Check sheet for the drawn part. Datum: minimum x, y, z corner. Units: mm. Round coordinates to 2 decimals unless told otherwise and drop trailing zeros. Write each loop counter-clockwise with the first axis right and the second up, starting at its lowest first coordinate (ties: lowest second). Pieces come first, ordered by that corner, then holes.
Item 1: Cross-section at A-A on z = 161. Enter the section's corners in (x, y).
Item 2: Material ranges on line 1 (X direction, y = 2.55, z = 169); line 2 (Z direction, x = 19.5, y = 2.7), recorded low to high.
Item 3: Go/stop test with flat-tipped pins: pin 1 Ø1.5 at (x, y) = (75.5, 2) entering from +Z; pin 2 Ø1.5 at (y, z) = (2, 165) entering from -X; pin 3 Ø4 at (x, z) = (132, 134.5) entering from +Y; pin 4 Ø8 at (x, z) = (129, 112) entering from -Y. Record where each tip stops, or that it passes through.
Item 4: Cross-section at B-B on y = 1.3. Enter the section's corners in (x, z), plus the area to 3 significant figures.
Item 5: Cross-section at C-C on x = 31.5. Enter the section's corners in (y, z), plus the area to 3 significant figures.
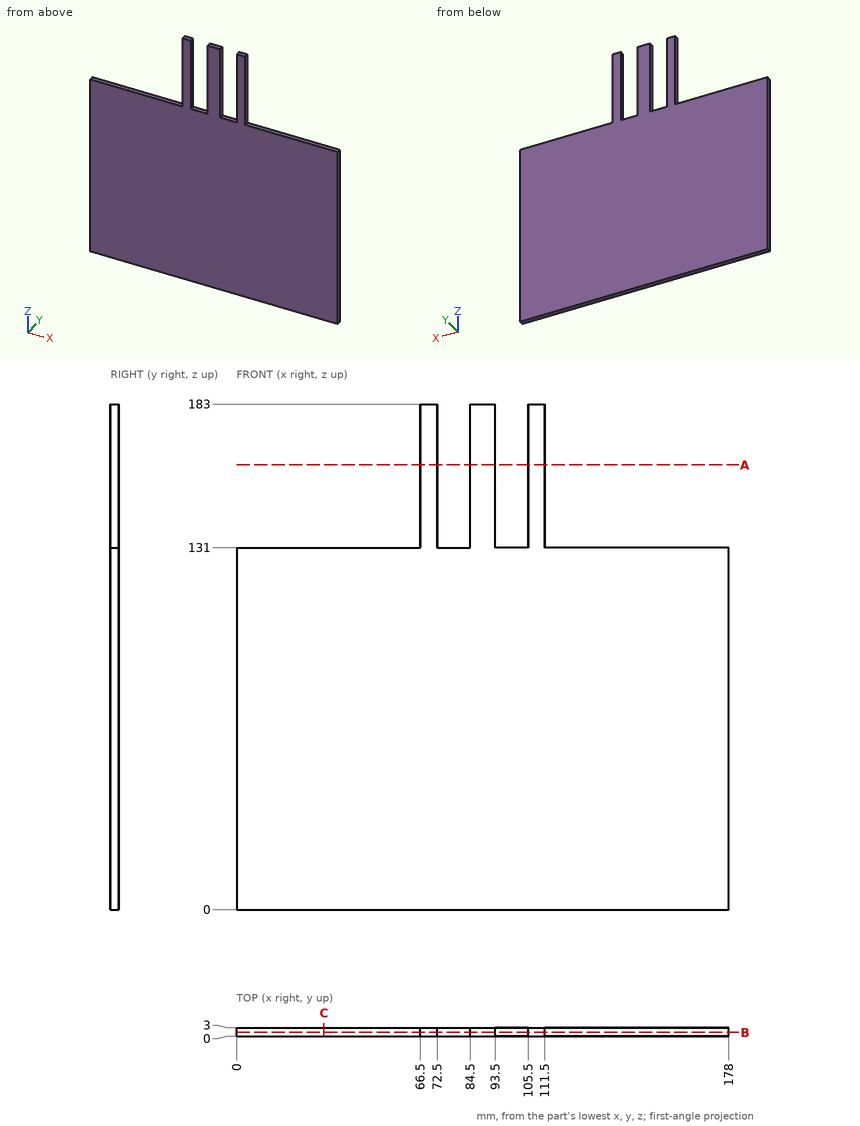
Response values:
1. outline: (66.5, 0) - (72.5, 0) - (72.5, 3) - (66.5, 3) - close; (84.5, 0) - (93.5, 0) - (93.5, 3) - (84.5, 3) - close; (105.5, 0) - (111.5, 0) - (111.5, 3) - (105.5, 3) - close
2. line 1: x = 66.5 to 72.5, 84.5 to 93.5, 105.5 to 111.5
2. line 2: z = 0 to 131
3. pin 1: stops at z = 131
3. pin 2: stops at x = 66.5
3. pin 3: passes through
3. pin 4: stops at y = 0
4. outline: (0, 0) - (178, 0) - (178, 131) - (111.5, 131) - (111.5, 183) - (105.5, 183) - (105.5, 131) - (93.5, 131) - (93.5, 183) - (84.5, 183) - (84.5, 131) - (72.5, 131) - (72.5, 183) - (66.5, 183) - (66.5, 131) - (0, 131) - close
4. area: 24,400 mm2
5. outline: (0, 0) - (3, 0) - (3, 131) - (0, 131) - close
5. area: 393 mm2
